Can you work these out from the model? Positions are in its coordinate system, mm. A direction names the side the tool comes from. Give positions to 0.01 mm unless a question says otherwise; leave off trailing zeros. Write each loop counter-clockwise with the first axis right and the second up, starting at its lowest first coordinate (ties: lowest second). Pieces come first, ordered by that corner, then holes. Notation, with made-up numbers: (39, 13) -> (91, 13) arc R20 ccw to (91, 35) -> close; hole circle Ø5 at (-8.5, 6.5). An arc over 180 degrees is marked (long way). Answer as CSV lines item,"result". Start each with the question number.
1. If we section it at B-B on y = 0: Write out the boundary of the cut face in (x, z) (1 decimal), plus the area to 3 significant figures.
2. If we section it at A-A on z = 21: Write out the boundary of the cut face in (x, y) (3 decimals).
3. I'm going to push flat-ended pins straight in: P1, Ø5.5, axis at x = -1.5, y = 1.5, coming from the +Z side; P2, Ø1.5, axis at x = 3, y = -3, coming from the +Z side; P3, Ø1.1, axis at y = -3, z = 34, coming from the +X side; P4, Ø0.5, axis at y = 0, z = 45, coming from the -X side (3 decimals). Where does each tip first touch, or does it pass through?
4. I need wall thicknesses on line 1 (Z direction, x = 4.25, y = -1.5); line 2 (X direction, y = 0, z = 19.5) (3 decimals); line 3 (X direction, y = -2.5, z = 24). Which ranges of each line are inside material? Lowest first, please. Write a range as [from, to].
5. On a 3-axis mill with a long thin cutter (end or side, diameter ignored), from which of +Z, -Z, +X, -X, +Y, -Y can I reach the whole of each face in a straight line? I mean faces 1 (the face through (0, 4.445, 36)), 2 (the face through (-0.889, 3, 36)), 3 (the face through (0.889, 3, 36)), 4 (the face through (-0.889, -3, 36)). Say none if no direction works.
```python
from build123d import *

# Parameters (mm, degrees)
F1_DEPTH = 73.66
F2_R     = 5.3975
F3_DEPTH = 1.778


with BuildPart() as f1:
    # F0 (on Top) → F1 (new body)
    with BuildSketch(Plane.XY):
        Polygon((0.889, 4.445), (-0.889, 4.445), (-0.889, 0.889), (-4.445, 0.889), (-4.445, -0.889), (-0.889, -0.889), (-0.889, -4.445), (0.889, -4.445), (0.889, -0.889), (4.445, -0.889), (4.445, 0.889), (0.889, 0.889), align=None)
    extrude(amount=F1_DEPTH)

    # F2 (on Top) → F3 (join)
    with BuildSketch(Plane.XY):
        Circle(F2_R)
    extrude(amount=-F3_DEPTH)


solid = f1.part
```
Computed values:
1,outline,"(-5.4, -1.8) -> (5.4, -1.8) -> (5.4, 0) -> (4.4, 0) -> (4.4, 73.7) -> (-4.4, 73.7) -> (-4.4, 0) -> (-5.4, 0) -> close"
1,area,"674 mm2"
2,outline,"(-4.445, -0.889) -> (-0.889, -0.889) -> (-0.889, -4.445) -> (0.889, -4.445) -> (0.889, -0.889) -> (4.445, -0.889) -> (4.445, 0.889) -> (0.889, 0.889) -> (0.889, 4.445) -> (-0.889, 4.445) -> (-0.889, 0.889) -> (-4.445, 0.889) -> close"
3,P1,"stops at z = 73.66"
3,P2,"stops at z = 0"
3,P3,"stops at x = 0.89"
3,P4,"stops at x = -4.445"
4,line 1,"z = [-1.78, 0]"
4,line 2,"x = [-4.445, 4.445]"
4,line 3,"x = [-0.89, 0.89]"
5,face 1,"+Z, +X, -X, +Y"
5,face 2,"+Z, -X, +Y"
5,face 3,"+Z, +X, +Y"
5,face 4,"+Z, -X, -Y"
